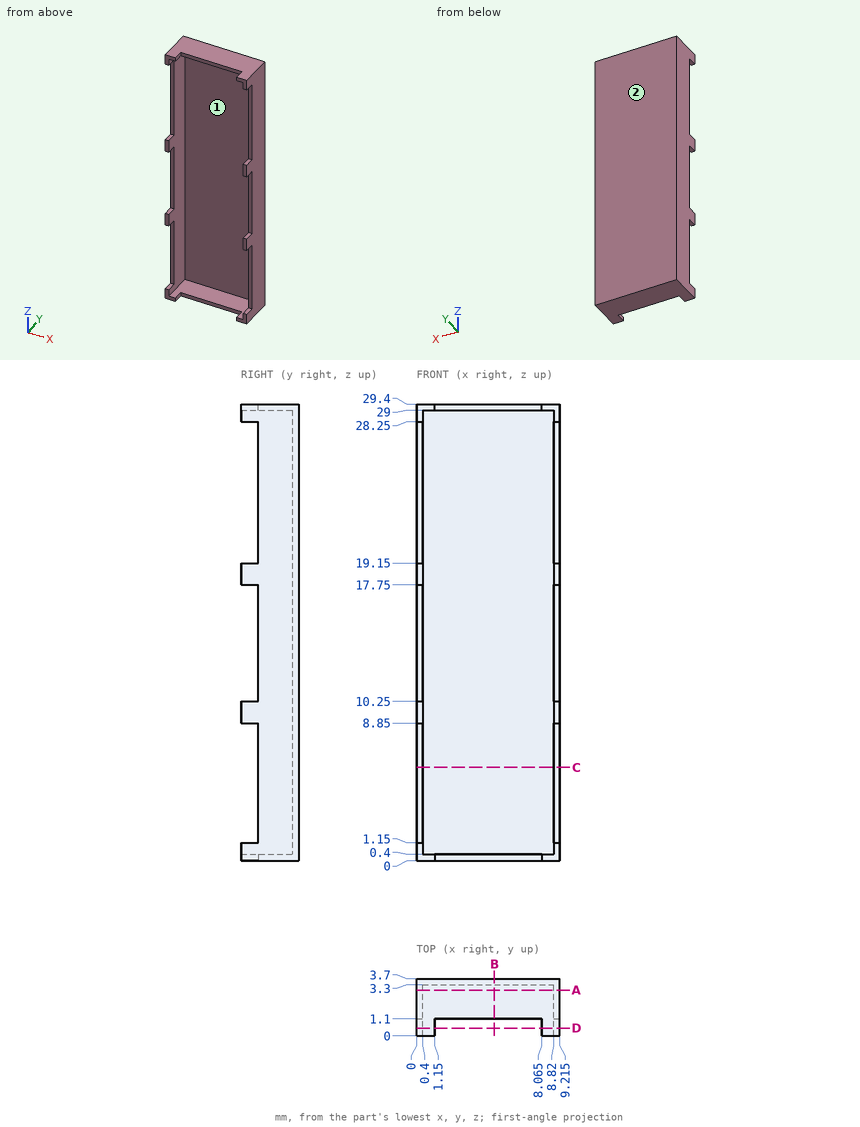
Job drawing, mm, ordinate dimensions from the low corner. One solid piece. Coordinates: 2 decimals unless noted, no trailing zeros. Order: outer loops, then holes, each group sorted by start corner. A loop starts at its lowest first (then second) coordinate and runs counter-clockwise, first axis right, second up. Notation, with made-up numbers: (-36, 17.25) -> (-19, 17.25) arc R28 ccw to (-19, 54.25) -> close; hole circle Ø1 at (-6, -23.75). An arc over 180 degrees is marked (long way). Answer in a Markdown table with one row per item. Add a question column.
Q1. Band-saw the part on D-D, the plane y = 0.5. Give the number of separate pieces and of enclosed holes in the cut face, then the cut area to 3 significant figures.
Q2. Band-saw the part on A-A, the plane y = 2.95. List the corners of the cut face in (x, z) (3 decimals).
Q3. Band-saw the part on B-B, the plane x = 5. List the corners of the cut face in (y, z).
Q4. Mould opens along X. For the marked faces 1 and 2 say: +X half, -X half, draft (parallel to the pull), parting line (faces both ways), or undercut.
Q5. Band-saw the part on C-C, the plane z = 6. List the corners of the cut face in (x, y) (3 decimals).
Q6. Wall check: line 1 along Z through (x, y) = (6.75, 2.95); line 2 along X through (y, z) = (2.4, 27.25) (3 decimals); line 3 along Y through (x, z) = (8.25, 25). Give the ranges that are in metal, low to high. Write a range as [from, to].
Q7. Drop flat-ended pins along their axis: pin 1 (4 mm diameter, centred on x = 2, z = 15, fed in from -Y); pin 2 (2.5 mm diameter, centred on x = 4.5, z = 20.5, fed in from -Y). Give the stop position or say it passes through.
Answers follow:
| question | item | result |
|---|---|---|
| 1 | separate pieces | 8 |
| 1 | enclosed holes | 0 |
| 1 | area | 5.26 mm^2 |
| 2 | outline | (0, 0) -> (9.215, 0) -> (9.215, 29.4) -> (0, 29.4) -> close; hole (0.4, 0.4) -> (8.82, 0.4) -> (8.82, 29) -> (0.4, 29) -> close |
| 3 | outline | (1.1, 0) -> (3.7, 0) -> (3.7, 29.4) -> (1.1, 29.4) -> (1.1, 29) -> (3.3, 29) -> (3.3, 0.4) -> (1.1, 0.4) -> close |
| 4 | face 1 | undercut |
| 4 | face 2 | draft |
| 5 | outline | (0, 1.1) -> (0.4, 1.1) -> (0.4, 3.3) -> (8.82, 3.3) -> (8.82, 1.1) -> (9.215, 1.1) -> (9.215, 3.7) -> (0, 3.7) -> close |
| 6 | line 1 | [0, 0.4], [29, 29.4] |
| 6 | line 2 | [0, 0.4], [8.82, 9.215] |
| 6 | line 3 | [3.3, 3.7] |
| 7 | pin 1 | y = 1.1 |
| 7 | pin 2 | y = 3.3 |
